Geometry: see drawing. Coordinates: mm, zero at the bounding-box minimum. A direction names the side the tool comes from. Give positions to 0.01 mm unless a question says otherwise; leave off trailing zeros. Write each loop counter-clockwise with the first axis right and the second up, starting at its lowest first coordinate (ties: lowest second). Pieces come first, ordered by that corner, then holes. Notation, with made-up numbers: (-4.75, 74) -> (35.25, 74) arc R28 cw to (35.25, 96) -> close; hole circle Ø9 at (-5.75, 42.5). An arc over 180 degrees is marked (long way). Use one line per item in the form item = value. Start each with the question number.
(1) Set-up query: the marked faces 1 and 2. Return all of +Z, -Z, +X, -X, +Y, -Y with unobstructed straight access to the full face (end or side cutting, diameter ignored); none if empty.
(2) Material intervals for line 1 along X through (y, z) = (2.65, 25.9); line 2 along Z through (x, y) = (36.85, 2.75); line 3 along Y through (x, z) = (20.5, 3), sorted ascending. Write a range as from..to.
(3) Cut plane D-D, the plane y = 14. Output: boundary loops of the cut face in (x, z), and give its area (3 significant figures).
(4) Cut plane B-B, the plane x = 4. Output: boundary loops of the cut face in (y, z).
(5) Cut plane C-C, the plane x = 25.9. Output: boundary loops of the cut face in (y, z), and give its area (3 significant figures).
(6) Cut plane A-A, the plane z = 25.9. Output: boundary loops of the cut face in (x, y).
(7) First-contact query: P1, Ø2.5, axis at x = 36.85, z = 6.93, coming from the -Y side; P2, Ø12, axis at y = 25.5, z = 15.5, coming from the -X side; P3, Ø5, axis at x = 13, z = 13.5, coming from the +Y side; P4, Ø3, axis at x = 26, y = 18, coming from the +Z side. Flat tips, straight axial feed; report the tip coordinate or a pass-through.
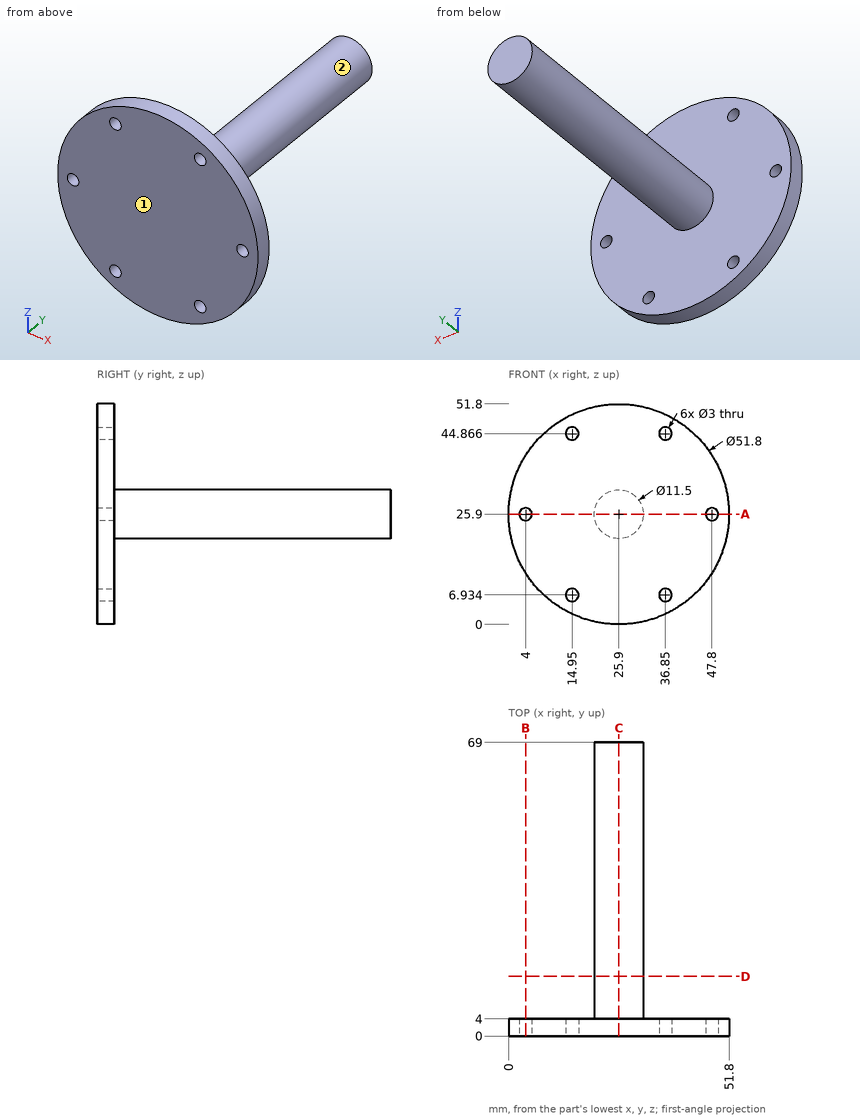
Geometry says:
q1.face_1 = +Z, -Z, +X, -X, -Y
q1.face_2 = +Y
q2.line_1 = 0..2.5, 5.5..46.3, 49.3..51.8
q2.line_2 = 2.43..5.43, 8.43..43.37, 46.37..49.37
q2.line_3 = 0..4
q3.outline = circle Ø11.5 at (25.9, 25.9)
q3.area = 104 mm^2
q4.outline = (0, 12.07) -> (4, 12.07) -> (4, 24.4) -> (0, 24.4) -> close; (0, 27.4) -> (4, 27.4) -> (4, 39.73) -> (0, 39.73) -> close
q5.outline = (0, 0) -> (4, 0) -> (4, 20.15) -> (69, 20.15) -> (69, 31.65) -> (4, 31.65) -> (4, 51.8) -> (0, 51.8) -> close
q5.area = 955 mm^2
q6.outline = (0, 0) -> (2.5, 0) -> (2.5, 4) -> (0, 4) -> close; (5.5, 0) -> (46.3, 0) -> (46.3, 4) -> (31.65, 4) -> (31.65, 69) -> (20.15, 69) -> (20.15, 4) -> (5.5, 4) -> close; (49.3, 0) -> (51.8, 0) -> (51.8, 4) -> (49.3, 4) -> close
q7.P1 = through
q7.P2 = 22.2
q7.P3 = 4
q7.P4 = 31.65
